CAD build for the part. Positions are in the model's coordinates, mm. A direction names the side the tool comes from. Coordinates: 2 decimals unless noted, no trailing zeros. Write each loop counter-clockwise with the first axis right and the second up, starting at its lowest first coordinate (ties: lowest second). Pieces come first, ordered by that corner, then holes.
Autodesk Inventor part; units mm, degrees
ref_plane "РабПлоскость1" through (33.5, -8.5, 0) normal (-1, 0, 0) x (0, 0, 1)
ref_plane "YZ Plane" through (0, 0, 0) normal (1, 0, 0) x (0, 1, 0)
ref_plane "XZ Plane" through (0, 0, 0) normal (0, 1, 0) x (-1, 0, 0)
sketch "Эскиз1" plane through (0, 0, 0) normal (0, 0, 1) x (1, 0, 0)
  line L0 (31.5, 14) -> (-48.5, 14)
  line L1 (-48.5, 14) -> (-48.5, -11)
  line L2 (-48.5, -11) -> (31.5, -11)
  line L3 (31.5, -11) -> (31.5, 14)
  line L4 (33.5, -8.5) -> (33.5, 11.5)
  point P0 (0, 0)
  point P1 (31.5, 1.5)
  point P2 (33.5, 1.5)
  dimension "d0" = 80
  dimension "d1" = 25
  dimension "d2" = 2
extrude "Выдавливание1" add sketch "Эскиз1" along normal blind 60
sketch "Эскиз2" plane through (-48.5, 14, 0) normal (0, 1, 0) x (1, 0, 0)
  line L0 (0, 0) -> (80, 0)
  line L1 (78, 0) -> (2, 0)
  line L2 (2, 0) -> (2, -58)
  line L3 (2, -58) -> (78, -58)
  line L4 (78, -58) -> (78, 0)
  line L5 (80, -60) -> (0, -60)
  line L6 (0, 0) -> (0, -60)
  line L7 (80, 0) -> (80, -60)
  point P0 (48.5, 0)
  dimension "d5" = 2
  dimension "d6" = 2
  dimension "d7" = 2
extrude "Выдавливание2" cut sketch "Эскиз2" against normal blind 23 contours L0 L4 L3 L2
sketch "Эскиз3" plane through (29.5, 14, 0) normal (-1, 0, 0) x (0, 0, 1)
  line L0 (58, 0) -> (58, -23)
  line L1 (0, -23) -> (58, -23)
  line L2 (58, -2) -> (0, -2)
  line L3 (0, -2) -> (0, -23)
  line L4 (0, -23) -> (58, -23)
  line L5 (58, -23) -> (58, -2)
  line L6 (0, 0) -> (58, 0)
  point P0 (0, -14)
  dimension "d10" = 2
ref_plane "РабПлоскость1" through (33.5, -8.5, 0) normal (-1, 0, 0) x (0, 0, 1)
extrude "Выдавливание3" cut sketch "Эскиз3" against normal up to surface (4 mm away)
properties part number "ДИ 00.00.07"
Item 1: Two-plate mould, pull along Y, no slides. Class faces 1 (the flat face through (-8, 14, 59)), 2 (the flat face through (30, 12, 29)), 3 (the flat face through (-46.5, 3, 29)): +Y half, -Y half, draft (parallel to the pull), parting line (faces both ways), or undercut.
Item 2: Wall check: line 1 along X through (y, z) = (9.75, 34); line 2 along Z through (x, y) = (25.5, -0.75); line 3 along Y through (x, z) = (-15, 51.5). Give the ranges that are in metal, low to high.
Item 3: Flat gauge pins, fed straight in: pin 1 Ø2 at (x, z) = (-17.5, 22.5) entering from +Y; pin 2 Ø1.5 at (y, z) = (-3.5, 13.5) entering from +X; pin 3 Ø11.5 at (x, y) = (4.5, 4) entering from -Z. Where does each tip first touch, or does it go through?
Item 4: Saw through at A-A, the plane z = 4. Write the cut outline in (x, y), and give its area (3 significant figures).
Item 5: Which spindle directions (+Z, -Z, +X, -X, +Y, -Y) get a long thin tool onto all of the face, cutting with end or side? Do faces 4 (the flat face through (30, 13, 0)), 5 (the flat face through (29.5, 13, 29)). Say none if no direction does.
Item 6: Saw through at B-B, the plane x = -21. Write the cut outline in (y, z), and give its area (3 significant figures).
Item 7: Saw through at C-C, the plane y = -6. Write the cut outline in (x, z).
Working result:
1. face 1: +Y half
1. face 2: undercut
1. face 3: draft
2. line 1: x = -48.5 to -46.5
2. line 2: z = 58 to 60
2. line 3: y = -11 to -9
3. pin 1: stops at y = -9
3. pin 2: stops at x = -46.5
3. pin 3: stops at z = 58
4. outline: (-48.5, -11) - (31.5, -11) - (31.5, -9) - (-46.5, -9) - (-46.5, 14) - (-48.5, 14) - close; (29.5, 12) - (31.5, 12) - (31.5, 14) - (29.5, 14) - close
4. area: 210 mm2
5. face 4: -Z, +X, -X, +Y, -Y
5. face 5: -Z, +Y
6. outline: (-11, 0) - (-9, 0) - (-9, 58) - (14, 58) - (14, 60) - (-11, 60) - close
6. area: 166 mm2
7. outline: (-48.5, 0) - (-46.5, 0) - (-46.5, 58) - (31.5, 58) - (31.5, 60) - (-48.5, 60) - close
